Autodesk Inventor part; units mm, degrees
ref_plane "YZ Plane" through (0, 0, 0) normal (1, 0, 0) x (0, 1, 0)
ref_plane "XZ Plane" through (0, 0, 0) normal (0, 1, 0) x (-1, 0, 0)
ref_plane "XY Plane" through (0, 0, 0) normal (0, 0, 1) x (1, 0, 0)
sketch "Sketch1" plane through (0, 0, 0) normal (0, 1, 0) x (-1, 0, 0)
  line L0 (-4, -15) -> (4, -15)
  line L1 (4, -15) -> (4, 15)
  line L2 (4, 15) -> (-4, 15)
  line L3 (-4, 15) -> (-4, -15)
  line L4 (-4, -15) -> (4, 15) construction
  line L5 (4, -15) -> (-4, 15) construction
  point P0 (0, 0)
  dimension "d0" = 8
  dimension "d1" = 30
extrude "Extrusion1" add sketch "Sketch1" along normal blind 3
sketch "Sketch3" plane through (0, 3, 0) normal (0, 1, 0) x (1, 0, 0)
  line L0 (-4, -15) -> (4, -15)
  line L1 (0, -15) -> (0, 15) construction
  line L2 (4, 15) -> (-4, 15)
  point P0 (0, 0)
  point P1 (0, -10)
  point P2 (0, 10)
  dimension "d8" = 5
  dimension "d9" = 5
hole "Hole1" at (0, 3, 10) at (0, 3, -10) direction (0, -1, 0) diameter 3.4 end through all
properties part number "turning clip top"
The model under review builds one solid part; all positions refer to its coordinate system, in mm. Round coordinates to 2 decimals unless told otherwise and drop trailing zeros. Loops run counter-clockwise (first coordinate to the right, second up) from the corner with the lowest first, then second, coordinate; pieces in that order, holes last. Notation, with made-up numbers: (79, 52.5) - (103, 52.5) arc R15 cw to (103, 74.5) - close; hole circle Ø1 at (9.5, 22.5). An arc over 180 degrees is marked (long way). Use a Markdown table: item, result. Add a question column.
Q1. The part is to be moulded in two halves that separate along X. For faces 1 (the face through (0.65, 1.48, -8.43)), 2 (the face through (0, 1, -15)), 3 (the face through (1.66, 1.48, 9.63)), 4 (the face through (-4, 1, 0)), say which applies: pulls with the +X half, pulls with the -X half, needs draft (parallel to the pull), parting line crosses it, or undercut.
Q2. Add section B-B (z = 10). State the section outline as (x, y) points.
Q3. Add section D-D (x = 1.25). State the section outline as (y, z) points.
Q4. Add section A-A (x = 0). State the section outline as (y, z) points.
Q5. For probe 1 along Z at (x, y) = (0, 0.7); probe 2 along X at (y, z) = (1.05, -10); probe 3 along Z at (x, y) = (1, 2.8), list the stretches that pass through material, from the lowest coordinate up.
Q6. Add section C-C (y = 0.9). State the section outline as (x, z) points, plus the area to 3 significant figures.
Worked answers:
| question | item | result |
|---|---|---|
| 1 | face 1 | undercut |
| 1 | face 2 | needs draft |
| 1 | face 3 | undercut |
| 1 | face 4 | pulls with the -X half |
| 2 | outline | (-4, 0) - (-1.7, 0) - (-1.7, 3) - (-4, 3) - close; (1.7, 0) - (4, 0) - (4, 3) - (1.7, 3) - close |
| 3 | outline | (0, -15) - (3, -15) - (3, -11.15) - (0, -11.15) - close; (0, -8.85) - (3, -8.85) - (3, 8.85) - (0, 8.85) - close; (0, 11.15) - (3, 11.15) - (3, 15) - (0, 15) - close |
| 4 | outline | (0, -15) - (3, -15) - (3, -11.7) - (0, -11.7) - close; (0, -8.3) - (3, -8.3) - (3, 8.3) - (0, 8.3) - close; (0, 11.7) - (3, 11.7) - (3, 15) - (0, 15) - close |
| 5 | probe 1 | -15 to -11.7, -8.3 to 8.3, 11.7 to 15 |
| 5 | probe 2 | -4 to -1.7, 1.7 to 4 |
| 5 | probe 3 | -15 to -11.37, -8.63 to 8.63, 11.37 to 15 |
| 6 | outline | (-4, -15) - (4, -15) - (4, 15) - (-4, 15) - close; hole circle Ø3.4 at (0, -10); hole circle Ø3.4 at (0, 10) |
| 6 | area | 222 mm² |
